The model under review builds one solid part; all positions refer to its coordinate system, in mm. Face numbers are marked on the shaded views. A direction names the side the tool comes from. Round coordinates to 2 decimals unless told otherwise and drop trailing zeros. Loops run counter-clockwise (first coordinate to the right, second up) from the corner with the lowest first, then second, coordinate; pieces in that order, holes last. Notation, with made-up numbers: (27.5, 37.5) -> (49.5, 37.5) arc R9 ccw to (49.5, 53.5) -> close; hole circle Ø7 at (67, 63). An arc over 180 degrees is marked (long way). Write each question's results on one line, items separated by ' | '. Start each with the question number.
Item 1: Mouldability with a two-part tool opening along X and no side actions: class the marked faces 1, 2 and 3 as pulls with the +X half, pulls with the -X half, needs draft (parallel to the pull), parting line crosses it, or undercut.
Item 2: Clearance check with flat-ended pins moving along their axes: pin 1 Ø1.5 at (x, z) = (20, 15.5) entering from +Y; pin 2 Ø0.9 at (x, z) = (-11, 14.5) entering from +Y; pin 3 Ø10 at (y, z) = (32, 10.5) entering from +X. State where each tip first meets the part, or that it passes through.
Item 3: We need section D-D (y = 20). Give the boundary of the cut face in (x, z), and give its area (3 significant figures).
Item 4: We need section C-C (x = 42). Give the boundary of the cut face in (y, z).
Item 5: We need section B-B (z = 5.75). Give the boundary of the cut face in (x, y).
Item 6: For L1, parallel to Y at x = 0, z = 22.15; L2, parallel to X at y = -10.7, z = 10; L3, parallel to Y at x = 0, z = 16.25, list the stretches that pass through material, from the lowest coordinate up. Write a range as from..to.
Item 7: We need section A-A (z = 10). Give the boundary of the cut face in (x, y).
Item 8: Tool access review of the marked faces 4 and 5: name each direction out of +Z, -Z, +X, -X, +Y, -Y from which nothing blocks a thin tool from reaching the whole face with its end or side.
from build123d import *

# Parameters (mm, degrees)
IZIM1_W                     = 20
IZIM1_H                     = 20
Y_KSEKLIK_EKSTR_ZYON1_DEPTH = 20
Y_KSEKLIK_EKSTR_ZYON2_DEPTH = 3
Y_KSEKLIK_EKSTR_ZYON3_DEPTH = 3
IZIM4_W                     = 26
IZIM4_H                     = 60
Y_KSEKLIK_EKSTR_ZYON4_DEPTH = 3
IZIM5_W                     = 63
IZIM5_H                     = 26
Y_KSEKLIK_EKSTR_ZYON5_DEPTH = 3
IZIM6_R                     = 7.5
KES_EKSTR_ZYON1_DEPTH       = 86.660287915
IZIM7_R                     = 2.5
KES_EKSTR_ZYON2_DEPTH       = 50
IZIM8_R                     = 1.924658324
IZIM8_R_2                   = 2.223723329
KES_EKSTR_ZYON3_DEPTH       = 50
IZIM9_R                     = 1.794605822
IZIM9_R_2                   = 1.816429962
KES_EKSTR_ZYON4_DEPTH       = 50


with BuildPart() as part:
    # Çizim1 → Yükseklik-Ekstrüzyon1 (new body)
    with BuildSketch(Plane.XY):
        Rectangle(IZIM1_W, IZIM1_H)
    extrude(amount=Y_KSEKLIK_EKSTR_ZYON1_DEPTH)

    # Çizim2 → Yükseklik-Ekstrüzyon2 (add)
    with BuildSketch(Plane.XY.offset(20)):
        Polygon((-10, -10), (-10, 10), (-10, 50), (-0.807466683, 57.713451316), (10, 57.713451316), (57.713451316, 10), (57.713451316, -0.807466683), (50, -10), (10, -10), align=None)
    extrude(amount=Y_KSEKLIK_EKSTR_ZYON2_DEPTH)

    # Çizim3 → Yükseklik-Ekstrüzyon3 (add)
    with BuildSketch(Plane(origin=(0, 0, 0), x_dir=(-1, 0, 0), z_dir=(0, 0, -1))):
        Polygon((10, -10), (-50, -10), (-57.713451316, -0.807466683), (-57.713451316, 10), (-10, 57.713451316), (0.807466683, 57.713451316), (10, 50), align=None)
    extrude(amount=Y_KSEKLIK_EKSTR_ZYON3_DEPTH)

    # Çizim4 → Yükseklik-Ekstrüzyon4 (add)
    with BuildSketch(Plane.ZY.offset(10)):
        with Locations((10, 20)):
            Rectangle(IZIM4_W, IZIM4_H)
    extrude(amount=Y_KSEKLIK_EKSTR_ZYON4_DEPTH)

    # Çizim5 → Yükseklik-Ekstrüzyon5 (add)
    with BuildSketch(Plane.XZ.offset(10)):
        with Locations((18.5, 10)):
            Rectangle(IZIM5_W, IZIM5_H)
    extrude(amount=Y_KSEKLIK_EKSTR_ZYON5_DEPTH)

    # Çizim6 → Kes-Ekstrüzyon1 (cut, through all)
    with BuildSketch(Plane.XY.offset(23)):
        Circle(IZIM6_R)
    extrude(amount=-KES_EKSTR_ZYON1_DEPTH, mode=Mode.SUBTRACT)

    # Çizim7 → Kes-Ekstrüzyon2 (cut)
    with BuildSketch(Plane(origin=(0, 0, -3), x_dir=(-1, 0, 0), z_dir=(0, 0, -1))):
        with Locations((-20, 0)):
            Circle(IZIM7_R)
        with Locations((-42, 0)):
            Circle(IZIM7_R)
        with Locations((0, 20)):
            Circle(IZIM7_R)
        with Locations((0, 42)):
            Circle(IZIM7_R)
    extrude(amount=-KES_EKSTR_ZYON2_DEPTH, mode=Mode.SUBTRACT)

    # Çizim8 → Kes-Ekstrüzyon3 (cut)
    with BuildSketch(Plane(origin=(-10, 0, 0), x_dir=(0, 0, -1), z_dir=(1, 0, 0))):
        with Locations(Location((-10, 20, 0), (0, 0, 90))):
            Circle(IZIM8_R)
        with Locations(Location((-10, 42, 0), (0, 0, 90))):
            Circle(IZIM8_R_2)
    extrude(amount=-KES_EKSTR_ZYON3_DEPTH, mode=Mode.SUBTRACT)

    # Çizim9 → Kes-Ekstrüzyon4 (cut)
    with BuildSketch(Plane(origin=(0, -10, 0), x_dir=(1, 0, 0), z_dir=(0, 1, 0))):
        with Locations(Location((20, -10, 0), (0, 0, 270))):
            Circle(IZIM9_R)
        with Locations(Location((42, -10, 0), (0, 0, 270))):
            Circle(IZIM9_R_2)
    extrude(amount=-KES_EKSTR_ZYON4_DEPTH, mode=Mode.SUBTRACT)


solid = part.part
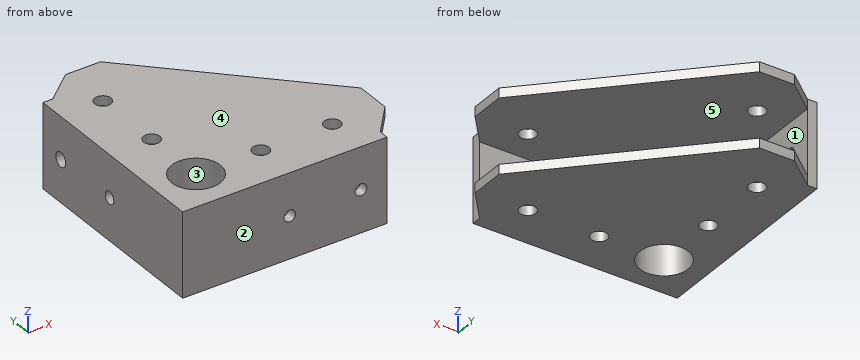
Here are the results:
1) face 1: pulls with the +X half | face 2: needs draft | face 3: undercut
2) pin 1: stops at y = -10 | pin 2: stops at y = 50 | pin 3: stops at x = -10
3) outline: (-13, -3) -> (-2.5, -3) -> (-2.5, 0) -> (-10, 0) -> (-10, 8.08) -> (-13, 8.08) -> close; (-13, 11.92) -> (-10, 11.92) -> (-10, 20) -> (-2.5, 20) -> (-2.5, 23) -> (-13, 23) -> close; (2.5, -3) -> (47.71, -3) -> (47.71, 0) -> (2.5, 0) -> close; (2.5, 20) -> (47.71, 20) -> (47.71, 23) -> (2.5, 23) -> close | area: 383 mm2
4) outline: (-13, -3) -> (-2.5, -3) -> (-2.5, 0) -> (-10, 0) -> (-10, 8.18) -> (-13, 8.18) -> close; (-13, 11.82) -> (-10, 11.82) -> (-10, 20) -> (-2.5, 20) -> (-2.5, 23) -> (-13, 23) -> close; (2.5, -3) -> (25.71, -3) -> (25.71, 0) -> (2.5, 0) -> close; (2.5, 20) -> (25.71, 20) -> (25.71, 23) -> (2.5, 23) -> close
5) outline: (-13, -13) -> (50, -13) -> (50, -10) -> (10, -10) -> (10, 10) -> (-10, 10) -> (-10, 50) -> (-13, 50) -> close; hole circle Ø15 at (0, 0)
6) L1: y = -13..-7.5, 7.5..17.5, 22.5..39.5, 44.5..57.71 | L2: x = -13..18.21, 21.79..40.18, 43.82..50 | L3: y = -13..-7.5, 7.5..10
7) outline: (-13, -13) -> (18.21, -13) -> (18.21, -10) -> (10, -10) -> (10, 10) -> (-10, 10) -> (-10, 18.08) -> (-13, 18.08) -> close; (-13, 21.92) -> (-10, 21.92) -> (-10, 39.78) -> (-13, 39.78) -> close; (-13, 44.22) -> (-10, 44.22) -> (-10, 50) -> (-13, 50) -> close; (21.79, -13) -> (40.18, -13) -> (40.18, -10) -> (21.79, -10) -> close; (43.82, -13) -> (50, -13) -> (50, -10) -> (43.82, -10) -> close; hole circle Ø15 at (0, 0)
8) face 4: +Z, +X, -X, +Y, -Y | face 5: +X, +Y
